Read the model definition and answer for the solid it produces. Units are mm, in the model's axes. A direction names the side the tool comes from. Give positions to 0.01 mm unless a question says otherwise; leave off trailing zeros. Write each loop counter-clockwise with the first axis right and the second up, starting at its lowest first coordinate (ties: lowest second). Pieces come first, ordered by that corner, then holes. Notation, with made-up numbers: (-25.75, 33.25) -> (10.25, 33.25) arc R32 ccw to (10.25, 63.25) -> close; hole circle Ø10 at (-27, 80.5). An arc over 180 degrees is marked (long way). Use a Markdown table: item, result.
from build123d import *

# Parameters (mm, degrees)
F1_DEPTH   = 20
F4_D       = 6.6
F4_ON_F3_D = 6.6


with BuildPart() as f1:
    # F0 (on Front) → F1 (new body, symmetric)
    with BuildSketch(Plane.XZ):
        Polygon((0, -47.9232184589), (-25, -47.9232184589), (-25, -49.9232184589), (2, -49.9232184589), (2, 213.0767815411), (27, 213.0767815411), (27, 215.0767815411), (0, 215.0767815411), align=None)
    extrude(amount=F1_DEPTH, both=True)

    # F4 (through all)
    with Locations(Plane.XY.offset(215.0767815411)):
        with Locations((13.5, 0)):
            Hole(F4_D / 2)

    # F4 on F3 (through all)
    with Locations(Plane.XY.offset(-47.9232184589)):
        with Locations((-12.5, 0)):
            Hole(F4_ON_F3_D / 2)


solid = f1.part
Item 1: A cutting plane is placed at B-B (x = 13.5). Give the vertices of the cut face in (y, z), then the cut area to 3 significant figures.
Return value:
| item | result |
|---|---|
| outline | (-20, 213.08) -> (-3.3, 213.08) -> (-3.3, 215.08) -> (-20, 215.08) -> close; (3.3, 213.08) -> (20, 213.08) -> (20, 215.08) -> (3.3, 215.08) -> close |
| area | 66.8 mm^2 |
Item 2: A cutting plane is placed at C-C (y = 10). Give the vertices of the cut face in (x, z), then the cut area to 3 significant figures.
Return value:
| item | result |
|---|---|
| outline | (-25, -49.92) -> (2, -49.92) -> (2, 213.08) -> (27, 213.08) -> (27, 215.08) -> (0, 215.08) -> (0, -47.92) -> (-25, -47.92) -> close |
| area | 630 mm^2 |
Item 3: A cutting plane is placed at A-A (y = 0). Give the vertices of the cut face in (x, z).
Return value:
| item | result |
|---|---|
| outline | (-25, -49.92) -> (-15.8, -49.92) -> (-15.8, -47.92) -> (-25, -47.92) -> close; (-9.2, -49.92) -> (2, -49.92) -> (2, 213.08) -> (10.2, 213.08) -> (10.2, 215.08) -> (0, 215.08) -> (0, -47.92) -> (-9.2, -47.92) -> close; (16.8, 213.08) -> (27, 213.08) -> (27, 215.08) -> (16.8, 215.08) -> close |
Item 4: A cutting plane is placed at D-D (x = -13.5). Give the vertices of the cut face in (y, z), then the cut area to 3 significant figures.
Return value:
| item | result |
|---|---|
| outline | (-20, -49.92) -> (-3.14, -49.92) -> (-3.14, -47.92) -> (-20, -47.92) -> close; (3.14, -49.92) -> (20, -49.92) -> (20, -47.92) -> (3.14, -47.92) -> close |
| area | 67.4 mm^2 |
Item 5: For a pull along Y with two mould halves and no side action, classify faces 4 (the face through (1, -20, 83)), 5 (the face through (0, 0, 85)), 6 (the face through (16.8, 0.1, 214.1)) as +Y half, -Y half, draft (parallel to the pull), parting line (faces both ways), or undercut.
Return value:
| item | result |
|---|---|
| face 4 | -Y half |
| face 5 | draft |
| face 6 | undercut |
Item 6: Each of these flat-tipped pins is pushed along its axis until it touches: P1, Ø8, axis at x = 8, y = -14.5, coming from the -Z side; P2, Ø5, axis at y = -4, z = 182.5, coming from the -X side; P3, Ø12, axis at y = -13.5, z = -2.5, coming from the +X side. Where does it stop, or does it pass through?
Return value:
| item | result |
|---|---|
| P1 | z = 213.08 |
| P2 | x = 0 |
| P3 | x = 2 |
Item 7: Straight lines are drawn through the part: line 1 along Y through (x, z) = (-12, -49); line 2 along X through (y, z) = (-2, -15.5); line 3 along Z through (x, y) = (22, -11.5). For each, find the intervals that lie inside material, in ascending order. Write a range as [from, to].
Return value:
| item | result |
|---|---|
| line 1 | [-20, -3.26], [3.26, 20] |
| line 2 | [0, 2] |
| line 3 | [213.08, 215.08] |
Item 8: A tool of negligible diameter and unlimited length cuts with its end or side. For faces 1 (the face through (-12, -5, -47.923)), 2 (the face through (-9.2, 0.1, -48.9)), 3 (the face through (17, 0, 213.077)), from which of +Z, -Z, +X, -X, +Y, -Y can it reach the whole face along a straight path? Write none if from no direction.
Return value:
| item | result |
|---|---|
| face 1 | +Z, -X, +Y, -Y |
| face 2 | +Z, -Z |
| face 3 | -Z, +X, +Y, -Y |
